Autodesk Inventor part; units mm, degrees
ref_plane "YZ Plane" through (0, 0, 0) normal (1, 0, 0) x (0, 1, 0)
ref_plane "XZ Plane" through (0, 0, 0) normal (0, 1, 0) x (-1, 0, 0)
ref_plane "XY Plane" through (0, 0, 0) normal (0, 0, 1) x (1, 0, 0)
sketch "スケッチ1" plane through (0, 0, 0) normal (0, 1, 0) x (-1, 0, 0)
  line L0 (0, 0) -> (35, 0)
  line L1 (35, 0) -> (35, -51)
  line L2 (35, -51) -> (0, -51)
  line L3 (0, -51) -> (0, 0)
  dimension "d0" = 35
  dimension "d1" = 51
extrude "押し出し1" add sketch "スケッチ1" along normal blind 10
sketch "スケッチ2" plane through (0, 10, 0) normal (0, 1, 0) x (1, 0, 0)
  line L0 (-35, 51) -> (-35, 0)
  line L1 (-35, 0) -> (0, 0)
  line L2 (-17.5, 0) -> (-17.5, 51)
  line L3 (0, 51) -> (-35, 51)
  line L4 (-35, 25.5) -> (0, 25.5)
  line L5 (0, 0) -> (0, 51)
  line L6 (-17.5, 25.5) -> (-27.65, 25.5)
  line L7 (-27.65, 25.5) -> (-27.65, 45.65)
  line L8 (-27.65, 45.65) -> (-17.5, 45.65)
  line L9 (-17.5, 45.65) -> (-17.5, 25.5)
  line L10 (-27.65, 25.5) -> (-27.65, 5.35)
  line L11 (-27.65, 5.35) -> (-17.5, 5.35)
  line L12 (-7.35, 25.5) -> (-7.35, 45.65)
  line L13 (-7.35, 45.65) -> (-17.5, 45.65)
  line L14 (-7.35, 25.5) -> (-7.35, 5.35)
  line L15 (-7.35, 5.35) -> (-17.5, 5.35)
  dimension "d7" = 20.15
  dimension "d8" = 10.15
extrude "押し出し2" add sketch "スケッチ2" along normal blind 40 contours L3 L2 L8 L7 L4 L0 | L4 L10 L11 L2 L1 L0 | L3 L5 L4 L12 L13 L2 | L2 L15 L14 L4 L5 L1
fillet "フィレット1" radius 5 4 edges at (0, 25, 0) (0, 25, -51) (-35, 25, -51) (-35, 25, 0)
sketch "スケッチ3" plane through (0, 0, -5) normal (1, 0, 0) x (0, 0, -1)
  line L0 (40.65, 50) -> (0.35, 50)
  line L1 (20.5, 50) -> (20.5, 0)
  line L2 (0, 0) -> (41, 0)
  line L3 (10.5, 50) -> (10.5, 0)
  line L4 (0, 50) -> (0, 0)
  line L5 (0, 10) -> (62, 10)
  line L6 (0.35, 10) -> (40.65, 10)
  point P0 (-5, 0)
  point P1 (10.5, 20)
  point P2 (10.5, 40)
  point P3 (30.5, 20)
  point P4 (30.5, 40)
  dimension "d12" = 10
  dimension "d13" = 10
  dimension "d14" = 10
  dimension "d15" = 20
hole "穴1" at (0, 20, -15.5) at (0, 40, -15.5) at (0, 40, -35.5) at (0, 20, -35.5) direction (-1, 0, 0) diameter 3.3 end through all
sketch "スケッチ4" plane through (-5, 0, -51) normal (0, 0, -1) x (-1, 0, 0)
  line L0 (0, 50) -> (0, 0)
  line L1 (0, 10) -> (25, 10)
  line L2 (25, 0) -> (25, 50)
  line L3 (0, 0) -> (25, 0)
  line L4 (2.35, 50) -> (22.65, 50)
  line L5 (12.5, 50) -> (12.5, 10)
  point P0 (-5, 0)
  point P1 (12.5, 20)
  point P2 (12.5, 40)
  dimension "d23" = 10
  dimension "d24" = 10
  dimension "d25" = 20
hole "穴2" at (-17.5, 20, -51) at (-17.5, 40, -51) direction (0, 0, 1) diameter 3.3 end through all
sketch "スケッチ5" plane through (0, 0, 0) normal (0, -1, 0) x (1, 0, 0)
  line L0 (-30, 0) -> (-5, 0)
  line L1 (-17.5, 0) -> (-17.5, -51)
  line L2 (-15.85, -51) -> (-19.15, -51)
  line L3 (0, -5) -> (0, -46)
  line L4 (0, -25.5) -> (-35, -25.5)
  line L5 (-35, -46) -> (-35, -5)
  point P0 (0, 0)
  point P1 (-17.5, -15.5)
  point P2 (-17.5, -35.5)
  dimension "d33" = 10
hole "穴3" at (-17.5, 0, -15.5) at (-17.5, 0, -35.5) direction (0, 1, 0) diameter 3.2 end through all
fillet "フィレット2" radius 1 4 edges at (-7.35, 50, -25.5) (-17.5, 50, -5.35) (-27.65, 50, -25.5) (-17.5, 50, -45.65)
sketch "スケッチ6" plane through (0, 0, 0) normal (0, -1, 0) x (1, 0, 0)
  line L0 (-27, -18.5) -> (-8, -18.5)
  line L1 (-8, -18.5) -> (-8, -32.5)
  line L2 (-8, -32.5) -> (-27, -32.5)
  line L3 (-27, -32.5) -> (-27, -18.5)
  circle A0 centre (-17.5, -15.5) radius 1.6
  circle A1 centre (-17.5, -35.5) radius 1.6
  line L4 (0, -5) -> (0, -46)
  line L5 (-35, -46) -> (-35, -5)
  point P0 (0, 0)
  dimension "d42" = 3
  dimension "d43" = 3
  dimension "d44" = 8
  dimension "d45" = 8
extrude "押し出し3" cut sketch "スケッチ6" against normal blind 10 contours L0 L1 L2 L3
properties part number "framefixpart2"
Part model, mm, in its own coordinate system. A direction names the side the tool comes from. Coordinates: 2 decimals unless noted, no trailing zeros. Order: outer loops, then holes, each group sorted by start corner. A loop starts at its lowest first (then second) coordinate and runs counter-clockwise, first axis right, second up.
(1) Tool access for faces 4 (the face through (-17.57, 38.35, -2.64)), 5 (the face through (-27.65, 29, -25)), 6 (the face through (-8, 5, -25)): list every direction of +Z, -Z, +X, -X, +Y, -Y with a clear straight run to the whole face (end or side of a thin tool).
Check sheet entries:
face 4: +Z, -Z
face 5: +Y
face 6: +Y, -Y
(2) Probe L1, parallel to Z at x = -17.5, y = 7.5; L2, parallel to Y at x = -1.75, z = -35.5; L3, parallel to Z at x = -6.5, y = 40. List the from-to ranges inside material, lowest first.
Check sheet entries:
L1: z = -51 to -37.1, -33.9 to -32.5, -18.5 to -17.1, -13.9 to 0
L2: y = 0 to 18.35, 21.65 to 38.35, 41.65 to 50
L3: z = -51 to -37.15, -33.85 to -17.15, -13.85 to 0
(3) Slice it at B-B, the plane z = -35.5. State how many separate pieces and enclosed holes the cut face has, and give its area (3 significant figures).
Check sheet entries:
separate pieces: 6
enclosed holes: 0
area: 809 mm2
(4) Slice it at D-D, the plane y = 6. Write the cut outline in (x, z), and give its area (3 significant figures).
Check sheet entries:
outline: (-35, -46) arc R5 ccw to (-30, -51) - (-5, -51) arc R5 ccw to (0, -46) - (0, -5) arc R5 ccw to (-5, 0) - (-30, 0) arc R5 ccw to (-35, -5) - close; hole (-27, -32.5) - (-8, -32.5) - (-8, -18.5) - (-27, -18.5) - close; hole circle Ø3.2 at (-17.5, -35.5); hole circle Ø3.2 at (-17.5, -15.5)
area: 1,480 mm2
(5) Slice it at A-A, the plane y = 14.5. Write the cut outline in (x, z), and give its area (3 significant figures).
Check sheet entries:
outline: (-35, -46) arc R5 ccw to (-30, -51) - (-5, -51) arc R5 ccw to (0, -46) - (0, -5) arc R5 ccw to (-5, 0) - (-30, 0) arc R5 ccw to (-35, -5) - close; hole (-27.65, -45.65) - (-7.35, -45.65) - (-7.35, -5.35) - (-27.65, -5.35) - close
area: 945 mm2
(6) Pin check, flat tip, straight feed: pin 1 Ø1 at (x, z) = (-18.5, -39) entering from +Y. Stop position of the tip, or through.
Check sheet entries:
pin 1: stops at y = 10
(7) Pull direction Z, two halves, no side cores. Call faces 1 (the face through (-18, 25, -51)), 2 (the face through (-6, 0, -25)), 3 (the face through (-31.38, 38.61, -16.39)): pulls with the +Z half, pulls with the -Z half, needs draft (parallel to the pull), parting line crosses it, or undercut.
Check sheet entries:
face 1: pulls with the -Z half
face 2: needs draft
face 3: undercut
